The drawing under review shows one solid part. Ordinate dimensions are in mm from its lowest x, y, z. Round coordinates to 2 decimals unless told otherwise and drop trailing zeros. Order: outer loops, then holes, each group sorted by start corner. A loop starts at its lowest first (then second) coordinate and runs counter-clockwise, first axis right, second up. Notation, with made-up numbers: M -18.75,64.25 L 31.25,64.25 A20 cw 31.25,102.25 Z; hole C 57.25,28.5 d1. An arc over 180 degrees is marked long. Answer as a JSON object with one key per item and string values. Group by question number.
1. Add section D-D on y = 3. State the section outline as (x, z) points.
2. Clearance check with a flat-ended pin moving along its axis: P1, Ø1.8, axis at x = 21, y = 5, coming from the +Z side. State where the tip first meets the part, or that it passes through.
3. Add section B-B on x = 21.5. State the section outline as (y, z) points (1 decimal).
4. Add section C-C on y = 5.5. State the section outline as (x, z) points (1 decimal).
5. Add section A-A on z = 0.8. Give the number of separate pieces and of enclosed holes in the cut face, and give its area (3 significant figures).
6. Mouldability with a two-part tool opening along X and no side actions: class the marked faces 1, 2, 3 and 4 as released by +X, released by -X, zero draft, split by the parting line, or undercut.
7. To check wall thickness, follow probe 1 along X at (y, z) = (5.75, 1.75) (1 decimal); probe 2 along X at (y, z) = (4, 0.2); probe 3 along Y at (x, z) = (21, 1.15). State the ranges of each line that lie inside material, in increasing order. Write a range as [from, to].
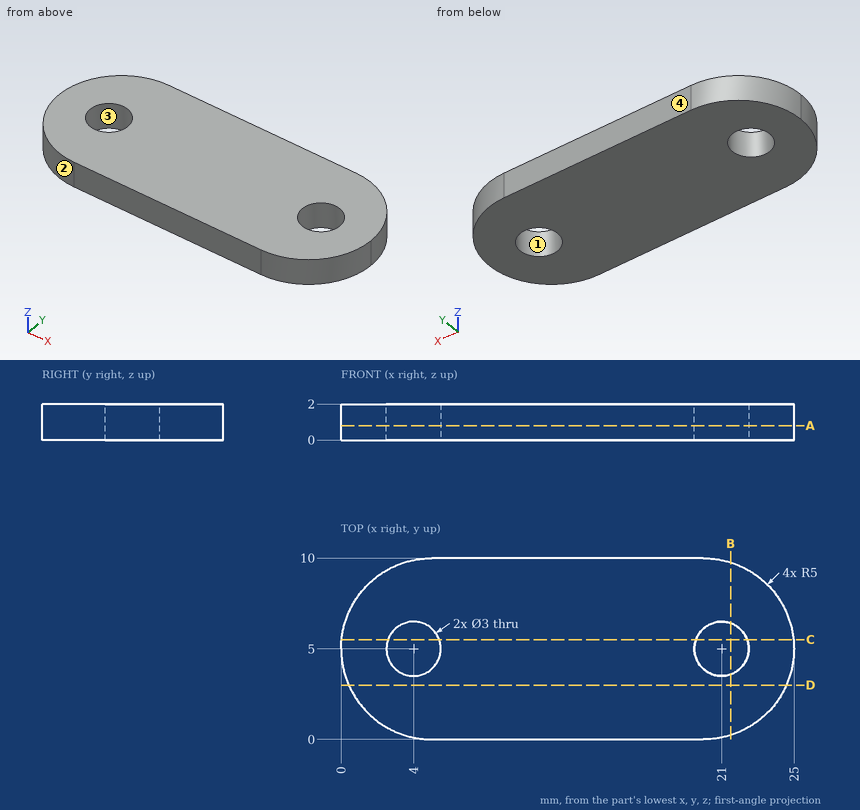
Recorded:
{
 "1": {"outline": "M 0.42,0 L 24.58,0 L 24.58,2 L 0.42,2 Z"},
 "2": {"P1": "passes through"},
 "3": {"outline": "M 0.2,0 L 3.6,0 L 3.6,2 L 0.2,2 Z; M 6.4,0 L 9.8,0 L 9.8,2 L 6.4,2 Z"},
 "4": {"outline": "M 0,0 L 2.6,0 L 2.6,2 L 0,2 Z; M 5.4,0 L 19.6,0 L 19.6,2 L 5.4,2 Z; M 22.4,0 L 25,0 L 25,2 L 22.4,2 Z"},
 "5": {"separate pieces": "1", "enclosed holes": "2", "area": "214 mm²"},
 "6": {"face 1": "undercut", "face 2": "released by -X", "face 3": "undercut", "face 4": "zero draft"},
 "7": {"probe 1": "x = [0.1, 2.7], [5.3, 19.7], [22.3, 24.9]", "probe 2": "x = [0.1, 2.88], [5.12, 19.88], [22.12, 24.9]", "probe 3": "y = [0.1, 3.5], [6.5, 9.9]"}
}
